The model under review builds one solid part; all positions refer to its coordinate system, in mm. Face numbers are marked on the shaded views. A direction names the side the tool comes from. Coordinates: 2 decimals unless noted, no trailing zeros. Write each loop counter-clockwise with the first axis right and the second up, starting at its lowest first coordinate (ties: lowest second). Pieces come first, ordered by that corner, then holes.
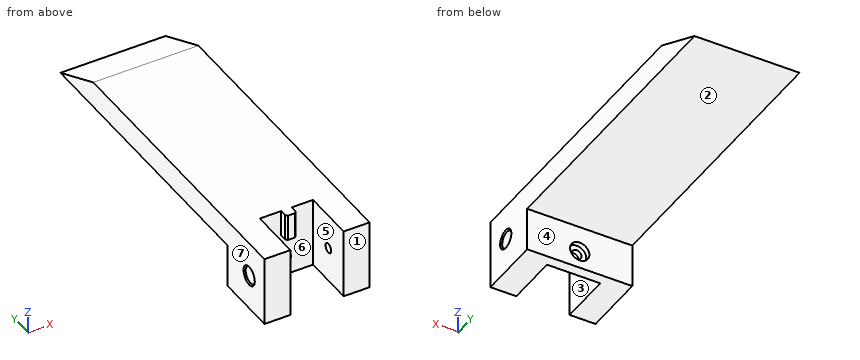
```python
from build123d import *

# Parameters (mm, degrees)
SKETCH_1_W                   = 30
SKETCH_1_H                   = 170
EXTRUDE_1_DEPTH              = 40
CUT_EXTRUDE_1_DEPTH          = 99.615414617
SKETCH_4_W                   = 25
SKETCH_4_H                   = 164
CUT_EXTRUDE_2_DEPTH          = 99.615414617
HOLE_WIZARD_M5_2_D           = 5.5
HOLE_WIZARD_M5_2_CBORE_D     = 11
HOLE_WIZARD_M5_2_CBORE_DEPTH = 3
SKETCH_9_W                   = 6
SKETCH_9_H                   = 15
EXTRUDE_2_DEPTH              = 5
CHAMFER_1_SIZE               = 1
EXTRUDE_3_DEPTH              = 15
SKETCH_11_W                  = 14.8
SKETCH_11_H                  = 40
EXTRUDE_4_DEPTH              = 30


with BuildPart() as part:
    # 스케치1 → 보스-돌출1 (new body)
    with BuildSketch(Plane.XY):
        Rectangle(SKETCH_1_W, SKETCH_1_H)
    extrude(amount=EXTRUDE_1_DEPTH)

    # 스케치3 → 컷-돌출1 (cut, through all)
    with BuildSketch(Plane(origin=(15, 0, 0), x_dir=(0, 0, -1), z_dir=(1, 0, 0))):
        Polygon((-40, 85), (-40, 52.832396192), (-25, 85), align=None)
    extrude(amount=-CUT_EXTRUDE_1_DEPTH, mode=Mode.SUBTRACT)

    # 스케치4 → 컷-돌출2 (cut, through all)
    with BuildSketch(Plane.ZY.offset(15)):
        with Locations((12.5, 3)):
            Rectangle(SKETCH_4_W, SKETCH_4_H)
    extrude(amount=-CUT_EXTRUDE_2_DEPTH, mode=Mode.SUBTRACT)

    # M5 소켓 머리 캡 나사용 카운터보어2 (through all)
    with Locations(Plane(origin=(0, -79, 0), x_dir=(1, 0, 0), z_dir=(0, 1, 0))):
        with Locations((0, -10)):
            CounterBoreHole(HOLE_WIZARD_M5_2_D / 2, HOLE_WIZARD_M5_2_CBORE_D / 2, HOLE_WIZARD_M5_2_CBORE_DEPTH)

    # 스케치9 → 보스-돌출2 (add)
    with BuildSketch(Plane.XZ.offset(85)):
        with Locations((0, 32.5)):
            Rectangle(SKETCH_9_W, SKETCH_9_H)
    extrude(amount=EXTRUDE_2_DEPTH)

    # 모따기1
    chamfer_1_edges = [part.edges().sort_by_distance(p)[0] for p in [
        (3, -90, 32.5),
        (-3, -90, 32.5),
    ]]
    chamfer(chamfer_1_edges, length=CHAMFER_1_SIZE)

    # 스케치10 → 보스-돌출3 (add)
    with BuildSketch(Plane.ZY.offset(15)):
        Polygon((25, -79), (0, -79), (0, -85), (40, -85), (40, 52.832396192), (25, 85), align=None)
    extrude_3 = extrude(amount=EXTRUDE_3_DEPTH)

    # 대칭 복사1: 보스-돌출3 across plane
    add(extrude_3.mirror(Plane.ZY))

    # 스케치11 → 보스-돌출4 (add)
    with BuildSketch(Plane.XZ.offset(85)):
        with Locations((-22.6, 20)):
            Rectangle(SKETCH_11_W, SKETCH_11_H)
        with Locations((22.6, 20)):
            Rectangle(SKETCH_11_W, SKETCH_11_H)
    extrude(amount=EXTRUDE_4_DEPTH)

    # 스케치14 → M5 소켓 머리 캡 나사용 카운터보어1 (revolve, cut)
    with BuildSketch(Plane(origin=(30, -100, 20), x_dir=(0, 0, -1), z_dir=(0, 1, 0))):
        Polygon((0, 0), (0, 14.8), (2.75, 14.8), (2.75, 12), (4.75, 12), (4.75, 0.75), (5.5, 0), align=None)
    hole_wizard_m5_1 = revolve(axis=Axis((36.35, -100, 20), (-1, 0, 0)), mode=Mode.SUBTRACT)

    # 대칭 복사2: M5 소켓 머리 캡 나사용 카운터보어1 across plane
    add(hole_wizard_m5_1.mirror(Plane.ZY), mode=Mode.SUBTRACT)


solid = part.part
```
Item 1: For pin 1 (15 mm diameter, centred on y = -97, z = 24.5, fed in from +X); pin 2 (6.5 mm diameter, centred on x = 0, z = 10, fed in from +Y); pin 3 (6 mm diameter, centred on x = -12, y = 49, fed in from -Z); pin 4 (2 mm diameter, centred on x = -13, z = 20, fed in from -Y), all flat-tipped, find the tip position at first contact; note any pin that passes through.
Solved:
pin 1: stops at x = 30
pin 2: stops at y = -82
pin 3: stops at z = 25
pin 4: stops at y = -85
Item 2: Take a section at D-D, the plane x = -11.5. Write out the cut boundary in (y, z), plus the area to 3 significant figures.
Solved:
outline: (-85, 0) - (-79, 0) - (-79, 25) - (85, 25) - (52.83, 40) - (-85, 40) - close
area: 2,460 mm2
Item 3: Machinability: for the marked faces 1, 2 and 3, which of the approach directions +Z, -Z, +X, -X, +Y, -Y give a long, thin tool a straight path to every point of the face, cutting with its end or side? Answer none if there is none.
Solved:
face 1: +Z, -Z, +X, -X, -Y
face 2: -Z, +X, -X, +Y
face 3: +Z, -Z, -Y
Item 4: Mouldability with a two-part tool opening along X and no side actions: class the marked faces 4, 5, 6 and 7 as pulls with the +X half, pulls with the -X half, needs draft (parallel to the pull), parting line crosses it, or undercut.
Solved:
face 4: needs draft
face 5: undercut
face 6: undercut
face 7: pulls with the -X half
Item 5: To check wall thickness, follow line 1 along Z through (x, y) = (25.75, -100); line 2 along Y through (x, z) = (-27, 19.5); line 3 along Z through (x, y) = (-16.8, -100). State the ranges of each line that lie inside material, in increasing order.
Solved:
line 1: z = 0 to 15.25, 24.75 to 40
line 2: y = -115 to -104.72, -95.28 to -79
line 3: z = 0 to 17.25, 22.75 to 40
Item 6: Take a section at A-A, the plane z = 10. Write out the cut boundary in (x, y).
Solved:
outline: (-30, -115) - (-15.2, -115) - (-15.2, -85) - (-2.75, -85) - (-2.75, -82) - (-5.5, -82) - (-5.5, -79) - (-30, -79) - close; (2.75, -85) - (15.2, -85) - (15.2, -115) - (30, -115) - (30, -79) - (5.5, -79) - (5.5, -82) - (2.75, -82) - close
Item 7: Take a section at B-B, the plane z = 20. Write out the cut boundary in (x, y).
Solved:
outline: (-30, -115) - (-15.2, -115) - (-15.2, -102.75) - (-18, -102.75) - (-18, -104.75) - (-29.25, -104.75) - (-30, -105.5) - close; (-30, -94.5) - (-29.25, -95.25) - (-18, -95.25) - (-18, -97.25) - (-15.2, -97.25) - (-15.2, -85) - (15.2, -85) - (15.2, -97.25) - (18, -97.25) - (18, -95.25) - (29.25, -95.25) - (30, -94.5) - (30, -79) - (-30, -79) - close; (15.2, -115) - (30, -115) - (30, -105.5) - (29.25, -104.75) - (18, -104.75) - (18, -102.75) - (15.2, -102.75) - close
Item 8: Take a section at C-C, the plane y = -100. Write out the cut boundary in (x, z), plus the area to 3 significant figures.
Solved:
outline: (-30, 0) - (-15.2, 0) - (-15.2, 17.25) - (-18, 17.25) - (-18, 15.25) - (-29.25, 15.25) - (-30, 14.5) - close; (-30, 25.5) - (-29.25, 24.75) - (-18, 24.75) - (-18, 22.75) - (-15.2, 22.75) - (-15.2, 40) - (-30, 40) - close; (15.2, 0) - (30, 0) - (30, 14.5) - (29.25, 15.25) - (18, 15.25) - (18, 17.25) - (15.2, 17.25) - close; (15.2, 22.75) - (18, 22.75) - (18, 24.75) - (29.25, 24.75) - (30, 25.5) - (30, 40) - (15.2, 40) - close
area: 924 mm2
